Can you work these out from the model? Positions are in its coordinate system, mm. Round coordinates to 2 decimals unless told otherwise and drop trailing zeros. Loops run counter-clockwise (first coordinate to the right, second up) from the corner with the lowest first, then second, coordinate; pieces in that order, holes last. Notation, with made-up numbers: M 5.25,-29 L 16.25,-29 A8 ccw 16.25,-18 Z; hole C -14.5,67.25 d2. An arc over 180 degrees is marked long. Return JSON: item names as keys, results as strings.
Autodesk Inventor part; units mm, degrees
ref_plane "cp_XY" through (2.5, 0, 0) normal (1, 0, 0) x (0, 0, -1)
ref_plane "cp_YZ" through (2.5, 0, 0) normal (0, 0, -1) x (0, 1, 0)
ref_plane "cp_ZX" through (2.5, 0, 0) normal (0, 1, 0) x (1, 0, 0)
sketch "Sketch_1" plane through (0, 0, 0) normal (0, 0, 1) x (1, 0, 0)
  line L0 (2.5, 0) -> (-2.5, 0)
  line L1 (-2.5, 0) -> (-2.5, 5)
  line L2 (-2.5, 5) -> (-2.067, 5.75)
  line L3 (-2.067, 5.75) -> (2.5, 5.75)
  line L4 (2.5, 5.75) -> (2.5, 0)
  line L5 (2.5, 0) -> (-2.5, 0)
revolve "Revolution1" add sketch "Sketch_1" angle 360 about axis through (2.5, 0, 0) along (1, 0, 0)
sketch "Sketch_2" plane through (0, 0, 0) normal (0, 0, 1) x (1, 0, 0)
  line L0 (2.5, 0) -> (-2.5, 0)
  line L1 (-2.5, 0) -> (-2.5, 3)
  line L2 (-2.5, 3) -> (-1.9585, 2.4585)
  line L3 (-1.9585, 2.4585) -> (1.9585, 2.4585)
  line L4 (1.9585, 2.4585) -> (2.5, 3)
  line L5 (2.5, 3) -> (2.5, 0)
  line L6 (2.5, 0) -> (-2.5, 0)
revolve "Revolution2" cut sketch "Sketch_2" angle 360 about axis through (2.5, 0, 0) along (1, 0, 0)
thread "Thread1"
sketch "Sketch_3" plane through (0, 0, 0) normal (1, 0, 0) x (0, 1, 0)
  line L0 (-10, 10) -> (-10, -10)
  line L1 (-10, -10) -> (10, -10)
  line L2 (10, -10) -> (10, 10)
  line L3 (10, 10) -> (-10, 10)
  line L4 (-2.8868, 5) -> (-5.7735, 0)
  line L5 (-5.7735, 0) -> (-2.8868, -5)
  line L6 (-2.8868, -5) -> (2.8868, -5)
  line L7 (2.8868, -5) -> (5.7735, 0)
  line L8 (5.7735, 0) -> (2.8868, 5)
  line L9 (2.8868, 5) -> (-2.8868, 5)
extrude "Extrusion1" cut sketch "Sketch_3" along normal mid plane 5
ref_plane "cp_XY" through (2.5, 0, 0) normal (1, 0, 0) x (0, 0, -1)
ref_plane "cp_YZ" through (2.5, 0, 0) normal (0, 0, -1) x (0, 1, 0)
ref_plane "cp_ZX" through (2.5, 0, 0) normal (0, 1, 0) x (1, 0, 0)
ref_plane "nut_to_screw_XY" through (0, 0, 0) normal (1, 0, 0) x (0, 0, -1)
ref_plane "nut_to_screw_YZ" through (0, 0, 0) normal (0, 0, -1) x (0, 1, 0)
ref_plane "nut_to_screw_ZX" through (0, 0, 0) normal (0, 1, 0) x (1, 0, 0)
properties part number "SLBNR6"
Q1. Suppose I cut it at A-A, the plane x = -0.4. Please give me the cut outline in (y, z).
Results:
{"outline": "M -5.75,-0.04 L -2.91,-4.96 A5.75 ccw -2.84,-5 L 2.84,-5 A5.75 ccw 2.91,-4.96 L 5.75,-0.04 A5.75 ccw 5.75,0.04 L 2.91,4.96 A5.75 ccw 2.84,5 L -2.84,5 A5.75 ccw -2.91,4.96 L -5.75,0.04 A5.75 ccw Z; hole C 0,0 d4.92"}
Q2. If I drill on line 1 along Z through (x, y) = (-0.3, 0); line 2 along Z through (x, y) = (-2.05, 1.5); line 3 along Y through (x, z) = (-0.95, 0.75), over which ranges is the centre line in solid material (lowest first)?
Results:
{"line 1": "z = -5 to -2.46, 2.46 to 5", "line 2": "z = -5 to -2.06, 2.06 to 5", "line 3": "y = -5.34 to -2.34, 2.34 to 5.34"}
Q3. Thinking about a two-plate mould opening in Z: for faces 1 (the flat face through (-0.035, 4.35, 2.466)), 2 (the cylindrical face through (0.027, 2.345, 0.738)), 3 (the conical face through (-2.38, 5.21, -0.11)), 4 (the flat face through (-2.5, 3.3, 0.1)), which applies, pulls with the +Z half, pulls with the -Z half, needs draft (parallel to the pull), parting line crosses it, or undercut?
Results:
{"face 1": "pulls with the +Z half", "face 2": "undercut", "face 3": "parting line crosses it", "face 4": "needs draft"}
